```python
from build123d import *

# Parameters (mm, degrees)
BOSS_EXTRUDE1_DEPTH = 7
CUT_EXTRUDE1_DEPTH  = 5.4


with BuildPart() as part:
    # Sketch1 → Boss-Extrude1 (new body)
    with BuildSketch(Plane(origin=(0, 0, 0), x_dir=(0, 1, 0), z_dir=(0, 0, 1))):
        with BuildLine():
            Line((-19.5, 15), (19.5, 15))
            ThreePointArc((19.5, 15), (25.156854249, 12.656854249), (27.5, 7))
            Line((27.5, 7), (27.5, -7))
            ThreePointArc((27.5, -7), (25.156854249, -12.656854249), (19.5, -15))
            Line((19.5, -15), (-19.5, -15))
            ThreePointArc((-19.5, -15), (-25.156854249, -12.656854249), (-27.5, -7))
            Line((-27.5, -7), (-27.5, 7))
            ThreePointArc((-27.5, 7), (-25.156854249, 12.656854249), (-19.5, 15))
        make_face()
    extrude(amount=BOSS_EXTRUDE1_DEPTH)

    # Sketch2 → Cut-Extrude1 (cut)
    with BuildSketch(Plane.XY.offset(7)):
        with BuildLine():
            Line((7, -25.9), (-7, -25.9))
            ThreePointArc((-7, -25.9), (-11.5254834, -24.0254834), (-13.4, -19.5))
            Line((-13.4, -19.5), (-13.4, 19.5))
            ThreePointArc((-13.4, 19.5), (-11.5254834, 24.0254834), (-7, 25.9))
            Line((-7, 25.9), (7, 25.9))
            ThreePointArc((7, 25.9), (11.5254834, 24.0254834), (13.4, 19.5))
            Line((13.4, 19.5), (13.4, -19.5))
            ThreePointArc((13.4, -19.5), (11.5254834, -24.0254834), (7, -25.9))
        make_face()
    extrude(amount=-CUT_EXTRUDE1_DEPTH, mode=Mode.SUBTRACT)


solid = part.part
```
Design review of the part built by this model. Coordinates are the model's own, in mm. A direction names the side the tool comes from. Round coordinates to 2 decimals unless told otherwise and drop trailing zeros. Write each loop counter-clockwise with the first axis right and the second up, starting at its lowest first coordinate (ties: lowest second). Pieces come first, ordered by that corner, then holes.
Item 1: The part is to be moulded in two halves that separate along Y. For faces 1 (the flat face through (0, 0, 0)), 2 (the cylindrical face through (-12.594, -25.219, 3.451)), 3 (the cylindrical face through (12.594, 25.219, 3.451)), 4 (the cylindrical face through (11.48, 24.07, 4.34)), say which applies: +Y half, -Y half, draft (parallel to the pull), parting line (faces both ways), or undercut.
Item 2: We need section B-B on y = -13. Write out the cut boundary in (x, z).
Item 3: For probe 1 along Y at (x, z) = (-6, 2); probe 2 along X at (y, z) = (7, 3.75); probe 3 along Z at (x, y) = (-10.5, 24), list the stretches that pass through material, from the lowest coordinate up.
Item 4: For faces 5 (the cylindrical face through (12.719, -25.094, 3.451)), 6 (the flat face through (0, -25.9, 4)), list the 3-axis set-ups (+Z, -Z, +X, -X, +Y, -Y) from which the entire face can be reached by the end or side of a thin tool; tool diameter is ignored.
Item 5: Clearance check with flat-ended pins moving along their axes: pin 1 Ø3 at (x, y) = (8.5, 21.5) entering from +Z; pin 2 Ø12 at (x, y) = (-1, 20.5) entering from -Z. State where each tip first meets the part, or that it passes through.
Item 6: We need section C-C on x = 0.5. Write out the cut boundary in (y, z).
Item 7: We need section A-A on z = 4.25. Write out the cut boundary in (x, y), and give its area (3 significant figures).
Returned:
1. face 1: draft
1. face 2: -Y half
1. face 3: +Y half
1. face 4: undercut
2. outline: (-15, 0) - (15, 0) - (15, 7) - (13.4, 7) - (13.4, 1.6) - (-13.4, 1.6) - (-13.4, 7) - (-15, 7) - close
3. probe 1: y = -27.5 to -25.9, 25.9 to 27.5
3. probe 2: x = -15 to -13.4, 13.4 to 15
3. probe 3: z = 0 to 1.6
4. face 5: +Z, -Z, +X, -Y
4. face 6: +Z
5. pin 1: stops at z = 1.6
5. pin 2: stops at z = 0
6. outline: (-27.5, 0) - (27.5, 0) - (27.5, 7) - (25.9, 7) - (25.9, 1.6) - (-25.9, 1.6) - (-25.9, 7) - (-27.5, 7) - close
7. outline: (-15, -19.5) arc R8 ccw to (-7, -27.5) - (7, -27.5) arc R8 ccw to (15, -19.5) - (15, 19.5) arc R8 ccw to (7, 27.5) - (-7, 27.5) arc R8 ccw to (-15, 19.5) - close; hole (-13.4, -19.5) arc R6.4 ccw to (-7, -25.9) - (7, -25.9) arc R6.4 ccw to (13.4, -19.5) - (13.4, 19.5) arc R6.4 ccw to (7, 25.9) - (-7, 25.9) arc R6.4 ccw to (-13.4, 19.5) - close
7. area: 242 mm2
